Design review of the part built by this model. Coordinates are the model's own, in mm. A direction names the side the tool comes from. Give positions to 0.01 mm unless a question says otherwise; leave off trailing zeros. Write each loop counter-clockwise with the first axis right and the second up, starting at its lowest first coordinate (ties: lowest second). Pieces come first, ordered by that corner, then holes. Notation, with made-up numbers: (61.25, 52) -> (79.25, 52) arc R29 ccw to (79.25, 85) -> close; hole circle Ø2 at (-30.75, -15.75). An arc over 180 degrees is marked (long way). Put each result on its own line as item: value. Start each with the question number.
Autodesk Inventor part; units mm, degrees
ref_plane "YZ Plane" through (0, 0, 0) normal (1, 0, 0) x (0, 1, 0)
ref_plane "XZ Plane" through (0, 0, 0) normal (0, 1, 0) x (-1, 0, 0)
ref_plane "XY Plane" through (0, 0, 0) normal (0, 0, 1) x (1, 0, 0)
sketch "Sketch1" plane through (0, 0, 0) normal (0, 1, 0) x (-1, 0, 0)
  line L0 (0, 0) -> (40, 0)
  line L1 (40, 0) -> (40, 14)
  line L2 (40, 14) -> (0, 14)
  line L3 (0, 14) -> (0, 0)
  dimension "d0" = 40
  dimension "d1" = 14
extrude "Extrusion1" add sketch "Sketch1" along normal blind 2
sketch "Sketch2" plane through (0, 2, 0) normal (0, 1, 0) x (1, 0, 0)
  line L0 (0, -14) -> (0, 0)
  line L1 (0, -11.242) -> (-5.5713, -11.242)
  line L2 (-5.5713, -11.242) -> (-5.5713, -2.1887)
  line L3 (-5.5713, -2.1887) -> (0, -2.1887)
  line L4 (0, -2.1887) -> (0, -11.242)
  line L5 (-38.2029, -11.242) -> (-36.4121, -11.242)
  line L6 (-36.4121, -11.242) -> (-36.4121, -2.1887)
  line L7 (-36.4121, -2.1887) -> (-38.2029, -2.1887)
  line L8 (-38.2029, -2.1887) -> (-38.2029, -11.242)
extrude "Extrusion2" add sketch "Sketch2" along normal blind 8
properties part number "00_LM286"
Q1. To check wall thickness, follow probe 1 along X at (y, z) = (3.5, 5.5); probe 2 along Y at (x, z) = (-26.5, 4.75); probe 3 along Z at (x, y) = (-5.5, 7.5). State the ranges of each line that lie inside material, in increasing order. Write a range as from..to.
Q2. Take a section at D-D on z = 13. Give the boundary of the cut face in (x, y).
Q3. Take a section at B-B on x = -4.5. Give the boundary of the cut face in (y, z), then the cut area to 3 significant figures.
Q4. Take a section at A-A on y = 5.25. Give the boundary of the cut face in (x, z), then the cut area to 3 significant figures.
Q5. Mouldability with a two-part tool opening along X and no side actions: class faces 1 (the face through (-20, 1, 14)), 2 (the face through (-5.571, 6, 7)), 3 (the face through (-40, 1, 7)), 4 (the face through (-20, 2, 7)) as +X half, -X half, draft (parallel to the pull), parting line (faces both ways), or undercut.
Q6. For pin 1 (4 mm diameter, centred on y = 4.5, z = 8.5, fed in from +X); pin 2 (4 mm diameter, centred on x = -6, y = 7.5, fed in from -Z); pin 3 (1.5 mm diameter, centred on x = -6.5, y = 7, fed in from -Z); pin 4 (1.7 mm diameter, centred on x = -2.5, y = 5, fed in from +Z), all flat-tipped, find the tip position at first contact; note any pin that passes through.
Q7. Take a section at C-C on z = 3. Give the boundary of the cut face in (x, y), then the cut area to 3 significant figures.
Q8. Machinability: for faces 5 (the face through (-37, 6, 11.242)), 6 (the face through (-37, 6, 2.189)), 7 (the face through (-38.203, 6, 7)), which of the approach directions +Z, -Z, +X, -X, +Y, -Y give a long, thin tool a straight path to every point of the face, cutting with its end or side? Answer none if there is none.
Result:
1. probe 1: x = -38.2..-36.41, -5.57..0
1. probe 2: y = 0..2
1. probe 3: z = 2.19..11.24
2. outline: (-40, 0) -> (0, 0) -> (0, 2) -> (-40, 2) -> close
3. outline: (0, 0) -> (2, 0) -> (2, 2.19) -> (10, 2.19) -> (10, 11.24) -> (2, 11.24) -> (2, 14) -> (0, 14) -> close
3. area: 100 mm^2
4. outline: (-38.2, 2.19) -> (-36.41, 2.19) -> (-36.41, 11.24) -> (-38.2, 11.24) -> close; (-5.57, 2.19) -> (0, 2.19) -> (0, 11.24) -> (-5.57, 11.24) -> close
4. area: 66.7 mm^2
5. face 1: draft
5. face 2: undercut
5. face 3: -X half
5. face 4: undercut
6. pin 1: stops at x = 0
6. pin 2: stops at z = 2.19
6. pin 3: passes through
6. pin 4: stops at z = 11.24
7. outline: (-40, 0) -> (0, 0) -> (0, 10) -> (-5.57, 10) -> (-5.57, 2) -> (-36.41, 2) -> (-36.41, 10) -> (-38.2, 10) -> (-38.2, 2) -> (-40, 2) -> close
7. area: 139 mm^2
8. face 5: +Z, +X, -X, +Y
8. face 6: -Z, +X, -X, +Y
8. face 7: +Z, -Z, -X, +Y
